```python
from build123d import *

# Parameters (mm, degrees)
F0_R     = 6
F1_DEPTH = 2
F2_SIZE2 = 2.5980762114
F2_SIZE  = 1.5
F4_R     = 2.5
F4_R_2   = 1.4
F5_DEPTH = 7
F6_R     = 1.2


# Not quite as in the source:
# - a fillet or chamfer that OpenCascade refuses, or shapes differently, is made with other operations: its cross-section is extruded or revolved along the edge and cut away or added


with BuildPart() as f1:
    # F0 (on Top) → F1 (new body)
    with BuildSketch(Plane.XY):
        Circle(F0_R)
    extrude(amount=F1_DEPTH)

    # F2
    f2_edges = [f1.edges().sort_by_distance(p)[0] for p in [
        (-6, 0, 0),
    ]]
    f2_side = f1.faces().sort_by_distance((-6, 0, 1))[0]
    chamfer(f2_edges, length=F2_SIZE, length2=F2_SIZE2, reference=f2_side)

    # F3: fillet of radius 1 on 2 edges, made by hand

    # F3_s1 → F3_t2 (revolve, cut)
    with BuildSketch(Plane.XZ):
        with BuildLine():
            ThreePointArc((3.6339745962, 0.1339745962), (3.3927936413, 0.0340741737), (3.1339745962, 0))
            Line((3.1339745962, 0), (3.4019237886, 0))
            Line((3.4019237886, 0), (3.6339745962, 0.1339745962))
        make_face()
    revolve(axis=Axis((0, 0, 0), (0, 0, 1)), mode=Mode.SUBTRACT)

    # F3_s3 → F3_t4 (revolve, cut)
    with BuildSketch(Plane.XZ):
        with BuildLine():
            ThreePointArc((6, 2), (5.8486778537, 1.5452494356), (5.5031382462, 1.2131367327))
            Line((5.5031382462, 1.2131367327), (6, 1.5))
            Line((6, 1.5), (6, 2))
        make_face()
    revolve(axis=Axis((0, 0, 1.5), (0, 0, 1)), mode=Mode.SUBTRACT)

    # F4 (on face) → F5 (join)
    with BuildSketch(Plane.XY.offset(2)):
        Circle(F4_R)
        Circle(F4_R_2, mode=Mode.SUBTRACT)
    extrude(amount=F5_DEPTH)

    # F6
    f6_edges = [f1.edges().sort_by_distance(p)[0] for p in [
        (-1.4, 0, 2),
    ]]
    fillet(f6_edges, radius=F6_R)


solid = f1.part
```
Build history of the part. All positions in model axes, mm. A direction names the side the tool comes from. Give positions to 0.01 mm unless a question says otherwise; leave off trailing zeros. Loops run counter-clockwise (first coordinate to the right, second up) from the corner with the lowest first, then second, coordinate; pieces in that order, holes last.
Item 1: Which spindle directions (+Z, -Z, +X, -X, +Y, -Y) get a long thin tool onto all of the face, cutting with end or side? Do faces 4 (the face through (1.1, -1.1, 9)), 5 (the face through (3, 0, 2)). Say none if no direction does.
Answers follow:
face 4: +Z, +X, -X, +Y, -Y
face 5: +Z
Item 2: Flat gauge pin, fed straight in: pin 1 (5 mm diameter, centred on y = 4, z = 8, fed in from -X). Where does the tip first touch, or does it go through?
Answers follow:
pin 1: stops at x = -2
Item 3: Slice it at A-A, the plane z = 7. List the corners of the cut face in (x, y).
Answers follow:
outline: circle Ø5 at (0, 0); hole circle Ø2.8 at (0, 0)
Item 4: Pull direction X, two halves, no side cores. Call faces 1 (the face through (-1.4, 0.06, 6.06)), 2 (the face through (-0.54, -2.44, 5.45)), 3 (the face through (0, 0, 0)): released by +X, released by -X, zero draft, split by the parting line, or undercut.
Answers follow:
face 1: undercut
face 2: split by the parting line
face 3: zero draft
Item 5: Drill centre lines: line 1 (Y direction, x = 0, z = 4.65); line 2 (Z direction, x = 1, y = 2.75); line 3 (Y direction, x = 0, z = 2.25). Where is each one in solid material? Low to high.
Answers follow:
line 1: y = -2.5 to -1.4, 1.4 to 2.5
line 2: z = 0 to 2
line 3: y = -2.5 to -0.93, 0.93 to 2.5
